Autodesk Inventor part; units mm, degrees
ref_plane "YZ Plane" through (0, 0, 0) normal (1, 0, 0) x (0, 1, 0)
ref_plane "XZ Plane" through (0, 0, 0) normal (0, 1, 0) x (-1, 0, 0)
ref_plane "XY Plane" through (0, 0, 0) normal (0, 0, 1) x (1, 0, 0)
sketch "Sketch1" plane through (0, 0, 0) normal (0, 0, 1) x (1, 0, 0)
  line L0 (114.3, 63.5) -> (-114.3, 63.5)
  line L1 (-114.3, 63.5) -> (-114.3, -63.5)
  line L2 (-114.3, -63.5) -> (114.3, -63.5)
  line L3 (114.3, -63.5) -> (114.3, 63.5)
  point P0 (0, 0)
  dimension "d0" = 228.6
  dimension "d1" = 127
extrude "Plate1" add sketch "Sketch1" along normal blind 3.048
sketch "Sketch2" plane through (0, 0, 3.048) normal (0, 0, 1) x (1, 0, 0)
  line L0 (-114.3, -63.5) -> (114.3, -63.5)
  line L1 (114.3, -63.5) -> (114.3, -60.325)
  line L2 (114.3, -63.5) -> (114.3, 63.5)
  line L3 (114.3, -60.325) -> (76.2, -60.325)
  line L4 (76.2, -60.325) -> (38.1, -60.325)
  line L5 (38.1, -60.325) -> (0, -60.325)
  line L6 (0, -60.325) -> (-38.1, -60.325)
  line L7 (-38.1, -60.325) -> (-76.2, -60.325)
  line L8 (-76.2, -60.325) -> (-114.3, -60.325)
  line L9 (-114.3, 63.5) -> (-114.3, -63.5)
  point P0 (0, 0)
  dimension "d3" = 3.175
  dimension "d4" = 38.1
  dimension "d5" = 38.1
  dimension "d6" = 38.1
  dimension "d7" = 38.1
hole "Hole1" at (-76.2, -60.325, 3.048) at (-38.1, -60.325, 3.048) at (0, -60.325, 3.048) at (38.1, -60.325, 3.048) at (76.2, -60.325, 3.048) direction (0, 0, -1) diameter 3.2766 depth 3.048
sketch "Sketch3" plane through (0, 0, 3.048) normal (0, 0, 1) x (1, 0, 0)
  line L0 (114.3, -63.5) -> (114.3, -25.4)
  line L1 (114.3, -63.5) -> (114.3, 63.5)
  line L2 (114.3, -25.4) -> (88.9, -25.4)
  line L3 (88.9, -25.4) -> (22.86, -25.4)
  line L4 (22.86, -25.4) -> (22.86, 2.54)
  line L5 (22.86, 2.54) -> (88.9, 2.54)
  line L6 (88.9, 2.54) -> (88.9, -25.4)
  point P0 (0, 0)
  dimension "d15" = 38.1
  dimension "d16" = 25.4
  dimension "d17" = 66.04
  dimension "d18" = 27.94
extrude "Cut1" cut sketch "Sketch3" against normal blind 3.048
sketch "Sketch4" plane through (0, 0, 3.048) normal (0, 0, 1) x (1, 0, 0)
  line L0 (114.3, 63.5) -> (-114.3, 63.5)
  line L1 (-114.3, 63.5) -> (-114.3, 50.8)
  line L2 (-114.3, -63.5) -> (-114.3, 63.5)
  line L3 (-114.3, 50.8) -> (-38.1, 50.8)
  line L4 (-38.1, 50.8) -> (38.1, 50.8)
  line L5 (38.1, 50.8) -> (114.3, 50.8)
  point P0 (0, 0)
  dimension "d21" = 12.7
  dimension "d22" = 76.2
  dimension "d23" = 76.2
  dimension "d24" = 76.2
hole "Hole2" at (-38.1, 50.8, 3.048) at (38.1, 50.8, 3.048) direction (0, 0, -1) diameter 2.1565 end through all
sketch "Sketch5" plane through (0, 0, 3.048) normal (0, 0, 1) x (1, 0, 0)
  circle A0 centre (-38.1, 50.8) radius 1.0782
  circle A1 centre (38.1, 50.8) radius 1.0782
  line L0 (22.86, 2.54) -> (88.9, 2.54)
  line L1 (88.9, 2.54) -> (88.9, -25.4)
  line L2 (88.9, -25.4) -> (22.86, -25.4)
  line L3 (22.86, -25.4) -> (22.86, 2.54)
  circle A2 centre (38.1, -60.325) radius 1.6383
  circle A3 centre (-38.1, -60.325) radius 1.6383
  circle A4 centre (-76.2, -60.325) radius 1.6383
  circle A5 centre (0, -60.325) radius 1.6383
  circle A6 centre (76.2, -60.325) radius 1.6383
  line L4 (114.3, 63.5) -> (114.3, -63.5)
  line L5 (-114.3, 63.5) -> (114.3, 63.5)
  line L6 (-114.3, -63.5) -> (-114.3, 63.5)
  line L7 (114.3, -63.5) -> (-114.3, -63.5)
  point P0 (0, 0)
hole "Hole3" at (22.86, 2.54, 3.048) at (88.9, 2.54, 3.048) at (88.9, -25.4, 3.048) at (22.86, -25.4, 3.048) direction (0, 0, -1) diameter 2.794 depth 3.048
sketch "Sketch6" plane through (0, 0, 3.048) normal (0, 0, 1) x (1, 0, 0)
  line L0 (114.3, -63.5) -> (-114.3, -63.5)
  line L1 (114.3, -63.5) -> (63.5, -63.5)
  line L2 (63.5, -63.5) -> (63.5, 25.4)
  point P0 (0, 0)
  dimension "d39" = 50.8
  dimension "d40" = 88.9
hole "Hole4" at (63.5, 25.4, 3.048) direction (0, 0, -1) diameter 6.7564 depth 3.048
equation "\"d13\" = Thickness"
equation "\"d19\" = Thickness"
equation "\"d37\" = Thickness"
equation "\"d46\" = Thickness"
equation "\"d2\" = Thickness"
equation "\"BendRadius\" = Thickness"
equation "\"BendReliefWidth\" = Thickness"
equation "\"BendReliefDepth\" = 0.5 * Thickness"
equation "\"CornerReliefSize\" = 4 * Thickness"
equation "\"MinimumRemnant\" = 2 * Thickness"
equation "\"TransitionRadius\" = BendRadius"
equation "\"JacobiRadiusSize\" = BendRadius"
equation "\"GapSize\" = Thickness"
properties part number "sheetmetalright2.0"
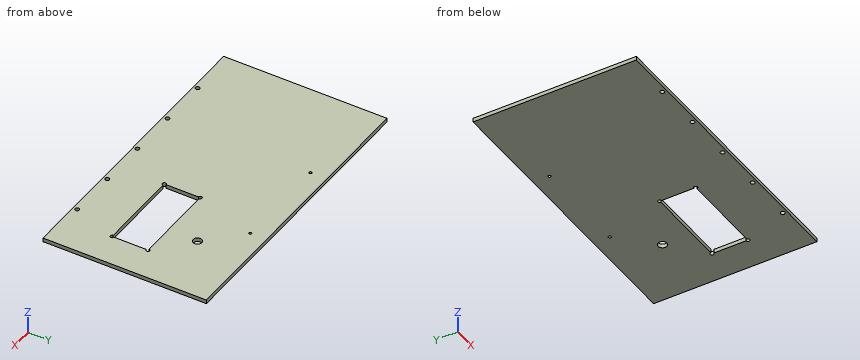
Model file for the job. Use its own axes, mm. Round coordinates to 2 decimals unless told otherwise and drop trailing zeros. Loops run counter-clockwise (first coordinate to the right, second up) from the corner with the lowest first, then second, coordinate; pieces in that order, holes last. Notation, with made-up numbers: M -0.75,-28 L 48.25,-28 A28 ccw 48.25,10 Z; hole C 13,83.25 d5. An arc over 180 degrees is marked long. Put each result on its own line as item: value. Start each with the question number.
Item 1: Cut at B-B (z = 0.95). Give the number of separate pieces and of enclosed holes in the cut face, then the cut area to 3 significant figures.
Item 2: Cut at D-D (y = 25.4). List the corners of the cut face in (x, z), then the cut area to 3 significant figures.
Item 3: Drill centre lines: line 1 along Y through (x, z) = (38.1, 2.15); line 2 along Y through (x, z) = (76.2, 2.1); line 3 along X through (y, z) = (25.4, 2.2). Where is each one in solid material? Low to high.
Item 4: Cut at A-A (y = -18). List the corners of the cut face in (x, z).
Item 5: Cut at C-C (x = 63.5). List the corners of the cut face in (y, z), then the cut area to 3 significant figures.
Item 6: Drop flat-ended pins along their axis: P1, Ø3, axis at x = 22.86, y = -25.4, coming from the +Z side; P2, Ø2, axis at x = 38.1, y = -60.325, coming from the -Z side. Give the stop position or say it passes through.
Answer block:
1. separate pieces: 1
1. enclosed holes: 9
1. area: 27,100 mm2
2. outline: M -114.3,0 L 60.12,0 L 60.12,3.05 L -114.3,3.05 Z; M 66.88,0 L 114.3,0 L 114.3,3.05 L 66.88,3.05 Z
2. area: 676 mm2
3. line 1: -63.5 to -61.96, -58.69 to -25.4, 2.54 to 49.72, 51.88 to 63.5
3. line 2: -63.5 to -61.96, -58.69 to -25.4, 2.54 to 63.5
3. line 3: -114.3 to 60.12, 66.88 to 114.3
4. outline: M -114.3,0 L 22.86,0 L 22.86,3.05 L -114.3,3.05 Z; M 88.9,0 L 114.3,0 L 114.3,3.05 L 88.9,3.05 Z
5. outline: M -63.5,0 L -25.4,0 L -25.4,3.05 L -63.5,3.05 Z; M 2.54,0 L 22.02,0 L 22.02,3.05 L 2.54,3.05 Z; M 28.78,0 L 63.5,0 L 63.5,3.05 L 28.78,3.05 Z
5. area: 281 mm2
6. P1: z = 3.05
6. P2: through
